Part model, mm, in its own coordinate system. A direction names the side the tool comes from. Round coordinates to 2 decimals unless told otherwise and drop trailing zeros. Loops run counter-clockwise (first coordinate to the right, second up) from the corner with the lowest first, then second, coordinate; pieces in that order, holes last.
from build123d import *

# Parameters (mm, degrees)
SKETCH4_OUTSIDE_W  = 15.138
SKETCH4_OUTSIDE_H  = 15.138
CUT_EXTRUDE1_DEPTH = 13.462
SKETCH6_OUTSIDE_W  = 22.586
SKETCH6_OUTSIDE_H  = 23.568
SKETCH6_OUTSIDE_R  = 2.54
CUT_EXTRUDE6_DEPTH = 2.54
CUT_EXTRUDE6_DRAFT = -60
CIRPATTERN3_COUNT  = 4


with BuildPart() as part:
    # Sketch3 → Revolve1 (revolve)
    with BuildSketch(Plane(origin=(0, 0, 0), x_dir=(0, 0, -1), z_dir=(1, 0, 0)), mode=Mode.PRIVATE) as revolve1_sk:
        Polygon((-12.7, 0), (12.7, 0), (12.7, 3.81), (-0.762, 3.81), (-0.762, 2.9591), (-12.7, 2.9591), align=None)
    revolve(revolve1_sk.sketch.rotate(Axis((0, 0, 12.7), (0, 0, -1)), 180), axis=Axis((0, 0, 12.7), (0, 0, -1)))

    # Sketch4 outside → Cut-Extrude1 (cut)
    with BuildSketch(Plane(origin=(0, 0, -12.7), x_dir=(-1, 0, 0), z_dir=(0, 0, -1))):
        Rectangle(SKETCH4_OUTSIDE_W, SKETCH4_OUTSIDE_H)
        Polygon((3.175, 1.833087105), (0, 3.666174209), (-3.175, 1.833087105), (-3.175, -1.833087105), (0, -3.666174209), (3.175, -1.833087105), align=None, mode=Mode.SUBTRACT)
    extrude(amount=-CUT_EXTRUDE1_DEPTH, mode=Mode.SUBTRACT)


with BuildPart() as cut_extrude6_tool:
    # Sketch6 outside → Cut-Extrude6 (with draft: the straight prism first)
    with BuildSketch(Plane(origin=(0, 0, -12.7), x_dir=(-1, 0, 0), z_dir=(0, 0, -1))):
        Rectangle(SKETCH6_OUTSIDE_W, SKETCH6_OUTSIDE_H)
        Circle(SKETCH6_OUTSIDE_R, mode=Mode.SUBTRACT)
    extrude(amount=-CUT_EXTRUDE6_DEPTH)
    # Cut-Extrude6: the draft: its side faces are tilted about the plane it starts from
    cut_extrude6_sides = [cut_extrude6_tool.faces().sort_by_distance(p)[0] for p in [
        (0, -11.784, -11.43),
        (-11.293, 0, -11.43),
        (0, 11.784, -11.43),
        (11.293, 0, -11.43),
        (2.54, 0, -11.43),
    ]]
    draft(cut_extrude6_sides, Plane(origin=(0, 0, -12.7), x_dir=(-1, 0, 0), z_dir=(0, 0, -1)), CUT_EXTRUDE6_DRAFT)


with BuildPart() as part_1:
    add(part.part)

    # Cut-Extrude6: cut by cut_extrude6_tool
    add(cut_extrude6_tool.part, mode=Mode.SUBTRACT)

    # Sketch12 → Cut-Revolve2 (revolve, cut)
    with BuildSketch(Plane(origin=(0, 0, 0), x_dir=(0, 0, -1), z_dir=(1, 0, 0))):
        Polygon((-0.762, 2.9591), (-0.762, 3.666174209), (-0.054925791, 3.666174209), align=None)
    revolve(axis=Axis((0, 0, 12.7), (0, 0, -1)), mode=Mode.SUBTRACT)

    # Cut-Sweep3: sweep along a path in Sketch10
    with BuildLine(Plane(origin=(0, 0, 0), x_dir=(0, 0, -1), z_dir=(0.7071067811865464, -0.7071067811865488, 0))) as cut_sweep3_path:
        ThreePointArc((-12.7, 0.898025612), (-8.161677229, 1.526035155), (-3.81, 2.9591))
    # Sketch7 → Cut-Sweep3 (sweep, cut)
    with BuildSketch(Plane.XY.offset(12.7)):
        with BuildLine():
            Line((0.635, 3.144163976), (0.635, 0.635))
            Line((0.635, 0.635), (3.144163976, 0.635))
            ThreePointArc((3.144163976, 0.635), (2.268148155, 2.268148155), (0.635, 3.144163976))
        make_face()
    cut_sweep3 = sweep(path=cut_sweep3_path.line, mode=Mode.SUBTRACT)

    # CirPattern3: Cut-Sweep3 ×4 about axis
    cirpattern3_axis = Axis((0, 0, 12.7), (0, 0, -1))
    for i in range(1, CIRPATTERN3_COUNT):
        add(cut_sweep3.rotate(cirpattern3_axis, i * 360 / CIRPATTERN3_COUNT), mode=Mode.SUBTRACT)

    # Sketch11 → Cut-Revolve1 (revolve, cut)
    with BuildSketch(Plane(origin=(0, 0, 0), x_dir=(1, 0, 0), z_dir=(0, 1, 0)), mode=Mode.PRIVATE) as cut_revolve1_sk:
        Polygon((1.27, -12.7), (2.9591, -8.128), (2.9591, -12.7), align=None)
    revolve(cut_revolve1_sk.sketch.rotate(Axis((0, 0, 12.7), (0, 0, -1)), 90), axis=Axis((0, 0, 12.7), (0, 0, -1)), mode=Mode.SUBTRACT)

    # Sketch13 → Cut-Revolve4 (revolve, cut)
    with BuildSketch(Plane(origin=(0, 0, 0), x_dir=(0, 0, -1), z_dir=(1, 0, 0))):
        Polygon((-12.7, 0.00254), (-12.46093948, 1.358319581), (-12.7, 1.358319581), align=None)
    revolve(axis=Axis((0, 0, 12.7), (0, 0, -1)), mode=Mode.SUBTRACT)

    # Sketch16 → Cut-Revolve5 (revolve, cut)
    with BuildSketch(Plane(origin=(0, 0, 0), x_dir=(0, 0, -1), z_dir=(1, 0, 0))):
        Polygon((4.7625, 3.666174209), (4.7625, 3.412174209), (5.3975, 3.666174209), align=None)
    revolve(axis=Axis((0, 0, 12.7), (0, 0, -1)), mode=Mode.SUBTRACT)


solid = part_1.part
1) Tool access for faces 1 (the face through (2.17, 0.02, 10.26)), 2 (the face through (1.133, -2.733, 3.678)): list every direction of +Z, -Z, +X, -X, +Y, -Y with a clear straight run to the whole face (end or side of a thin tool).
Values:
face 1: +Z, +X
face 2: +Z
2) Slice it at A-A, the plane z = -9. Give the cut face in (x, y) (3 decimals).
Values:
outline: (-3.175, -1.833) - (0, -3.666) - (3.175, -1.833) - (3.175, 1.833) - (0, 3.666) - (-3.175, 1.833) - close
3) Slice it at B-B, the plane z = -5. Give the cut face in (x, y) (3 decimals), then the cut area to 3 significant figures.
Values:
outline: (-3.175, -1.49) arc R3.507 ccw to (-2.878, -2.005) - (-0.297, -3.495) arc R3.507 ccw to (0.297, -3.495) - (2.878, -2.005) arc R3.507 ccw to (3.175, -1.49) - (3.175, 1.49) arc R3.507 ccw to (2.878, 2.005) - (0.297, 3.495) arc R3.507 ccw to (-0.297, 3.495) - (-2.878, 2.005) arc R3.507 ccw to (-3.175, 1.49) - close
area: 34.6 mm2
4) Drop flat-ended pins along their axis: pin 1 Ø0.6 at (x, y) = (3, -1.5) entering from -Z; pin 2 Ø3 at (x, z) = (-1, -4) entering from -Y. Give the stop position or say it passes through.
Values:
pin 1: stops at z = -12.4
pin 2: stops at y = -3.67
5) Wall check: line 1 along X through (y, z) = (2, -7.5); line 2 along Y through (x, z) = (1.75, 3.25); line 3 along Y through (x, z) = (1.5, -3.5). Give the ranges that are in metal, low to high.
Values:
line 1: x = -2.89 to 2.89
line 2: y = -2.39 to 2.39
line 3: y = -2.8 to 2.8
